Work out the finished part from the listing and answer in its coordinate system (mm). Coordinates: 2 decimals unless noted, no trailing zeros. Order: outer loops, then holes, each group sorted by start corner. A loop starts at its lowest first (then second) coordinate and runs counter-clockwise, first axis right, second up. Notation, with made-up numbers: (61, -27) -> (73, -27) arc R16 ccw to (73, -23) -> close; hole circle Ø6 at (21, 2). An arc over 180 degrees is marked (long way). Write item = value, one per line. Start each with the question number.
Q1. The part is cut by section B-B, the plane y = 1.6. Count the separate pieces of the cut face and the enclosed holes in it, plus the area to 3 significant figures.
Q2. The part is cut by section D-D, the plane x = -5.5. Determine the outline of the cut face in (y, z), plus the area to 3 significant figures.
Q3. Flat-ended cylindrical pins translate along their axes: pin 1 (3.5 mm diameter, centred on x = -25.86, z = -16.68, fed in from +Y); pin 2 (0.7 mm diameter, centred on y = 1, z = 8.5, fed in from +X). Find the tip coordinate at first contact, or state that the pin passes through.
Q4. Straight lines are drawn through the part: L1, parallel to Z at x = 25, y = 2.05; L2, parallel to Z at x = -26.5, y = 1.4; L3, parallel to Z at x = -25.5, y = 1.15. For each, find the intervals that lie inside material, in ascending order. Write a range as from..to.
Q5. The part is cut by section C-C, the plane z = 16. Determine the outline of the cut face in (x, y).
Q6. The part is cut by section A-A, the plane x = 26. Determine the outline of the cut face in (y, z), plus the area to 3 significant figures.
Autodesk Inventor part; units mm, degrees
ref_plane "YZ Plane" through (0, 0, 0) normal (1, 0, 0) x (0, 1, 0)
ref_plane "XZ Plane" through (0, 0, 0) normal (0, 1, 0) x (-1, 0, 0)
ref_plane "XY Plane" through (0, 0, 0) normal (0, 0, 1) x (1, 0, 0)
sketch "Sketch1" plane through (0, 0, 0) normal (0, 1, 0) x (-1, 0, 0)
  line L0 (38.4325, -41.9578) -> (13.0325, -41.9578)
  line L1 (13.0325, -41.9578) -> (13.0325, 27.6382)
  line L2 (13.0325, 27.6382) -> (38.4325, 27.6382)
  line L3 (38.4325, 27.6382) -> (38.4325, -41.9578)
  line L4 (38.4325, -41.9578) -> (-9.6784, 6.153) construction
  line L5 (38.4325, -41.9578) -> (38.4325, -16.5578)
  line L6 (38.4325, -16.5578) -> (-31.1635, -16.5578)
  line L7 (-31.1635, -16.5578) -> (-31.1635, -41.9578)
  line L8 (-31.1635, -41.9578) -> (38.4325, -41.9578)
  point P0 (0, 0)
  point P1 (13.0325, -16.5578)
  dimension "d0" = 25.4
  dimension "d1" = 69.596
  dimension "d2" = 45
extrude "Extrusion1" add sketch "Sketch1" along normal blind 2.286
chamfer "Chamfer1" distance 2.54 angle 45 1 edges at (-13.0325, 1.143, 27.6382)
chamfer "Chamfer2" distance 2.54 angle 45 4 edges at (-38.4325, 1.143, 27.6382) (31.1635, 1.143, -16.5578) (31.1635, 1.143, -41.9578) (-38.4325, 1.143, -41.9578)
fillet "Fillet1" radius 3.175 1 edges at (-13.0325, 1.143, -16.5578)
sketch "Sketch2" plane through (0, 2.286, 0) normal (0, 1, 0) x (1, 0, 0)
  circle A0 centre (-25.8595, 29.3848) radius 2.0828
  line L0 (28.6235, 41.9578) -> (-35.8925, 41.9578)
  line L1 (31.1635, 19.0978) -> (31.1635, 39.4178)
  point P0 (0, 0)
  dimension "d12" = 12.573
  dimension "d13" = 57.023
  dimension "d14" = 4.1656
extrude "Extrusion2" cut sketch "Sketch2" against normal blind 2.286
pattern_linear "Rectangular Pattern1" count 5 spacing 12.7 along (0, 0, 1) of "Extrusion2"
pattern_linear "Rectangular Pattern2" count 5 spacing 12.7 along (1, 0, 0) of "Extrusion2"
properties part number "VersaGusset 90o"
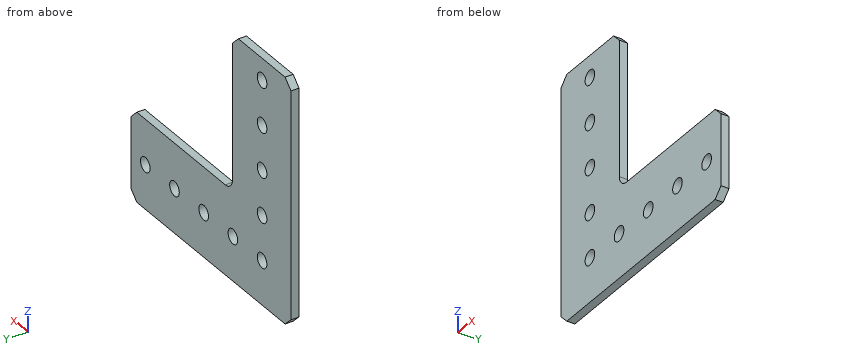
Model answer:
q1.separate_pieces = 1
q1.enclosed_holes = 9
q1.area = 2,750 mm2
q2.outline = (0, -41.96) -> (2.29, -41.96) -> (2.29, -16.56) -> (0, -16.56) -> close
q2.area = 58.1 mm2
q3.pin_1 = through
q3.pin_2 = -13.03
q4.L1 = -41.96..-31.47, -27.3..-16.56
q4.L2 = -41.96..-31.37, -27.4..-18.67, -14.7..-5.97, -2..6.73, 10.7..19.43, 23.4..27.64
q4.L3 = -41.96..-31.44, -27.33..-18.74, -14.63..-6.04, -1.93..6.66, 10.77..19.36, 23.47..27.64
q5.outline = (-38.43, 0) -> (-13.03, 0) -> (-13.03, 2.29) -> (-38.43, 2.29) -> close
q6.outline = (0, -41.96) -> (2.29, -41.96) -> (2.29, -31.18) -> (0, -31.18) -> close; (0, -27.59) -> (2.29, -27.59) -> (2.29, -16.56) -> (0, -16.56) -> close
q6.area = 49.9 mm2
